from build123d import *

# Parameters (mm, degrees)
F0_R     = 2.5
F1_DEPTH = 4
F2_SIZE  = 0.5


with BuildPart() as f1:
    # F0 (on Top) → F1 (new body)
    with BuildSketch(Plane.XY):
        Polygon((4, -2.309401), (4, 2.309401), (0, 4.618802), (-4, 2.309401), (-4, -2.309401), (0, -4.618802), align=None)
        Circle(F0_R, mode=Mode.SUBTRACT)
    extrude(amount=F1_DEPTH)

    # F2
    f2_edges = [f1.edges().sort_by_distance(p)[0] for p in [
        (-2.5, 0, 4),
        (-2.5, 0, 0),
    ]]
    chamfer(f2_edges, length=F2_SIZE)


solid = f1.part
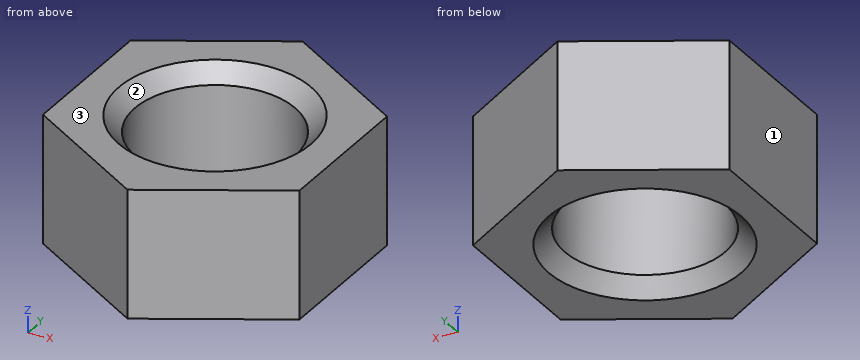
The model under review builds one solid part; all positions refer to its coordinate system, in mm. Face numbers are marked on the shaded views. Round coordinates to 2 decimals unless told otherwise and drop trailing zeros. Order: outer loops, then holes, each group sorted by start corner. A loop starts at its lowest first (then second) coordinate and runs counter-clockwise, first axis right, second up. Notation, with made-up numbers: (88, 48) -> (128, 48) arc R32 cw to (128, 80) -> close; hole circle Ø5 at (76, -19). An arc over 180 degrees is marked (long way). Use CSV: the item, a comma, the result in double quotes. Start each with the question number.
(1) Consider section B-B on z = 1.4. Write out the cut boundary in (x, y).
(2) Consider section C-C on x = 3.25. Write out the cut boundary in (y, z).
(3) Mouldability with a two-part tool opening along X and no side actions: class the marked faces 1, 2 and 3 as pulls with the +X half, pulls with the -X half, needs draft (parallel to the pull), parting line crosses it, or undercut.
(4) Consider section A-A on y = 0. Write out the cut boundary in (x, z).
(5) Wall thickness on probe 1 along X at (y, z) = (-2, 3.05); probe 2 along X at (y, z) = (-1, 3.2); probe 3 along Y at (x, z) = (-0.25, 1.2): over which ranges is each line inside the solid? List them lowest first. Write a range as from..to.
(6) Consider section D-D on y = 4. Write out the cut boundary in (x, z).
(7) Insertion check: pin 1 (1 mm diameter, centred on x = -2, z = 1, fed in from -Y); pin 2 (1 mm diameter, centred on y = 3.5, z = 0.5, fed in from +X); pin 3 (2 mm diameter, centred on x = -1, y = -1.5, fed in from +Z). Each pin has a flat end and moves straight along its axis. Give the tip position at first contact, or say it passes through.
Responses:
1,outline,"(-4, -2.31) -> (0, -4.62) -> (4, -2.31) -> (4, 2.31) -> (0, 4.62) -> (-4, 2.31) -> close; hole circle Ø5 at (0, 0)"
2,outline,"(-2.74, 0) -> (2.74, 0) -> (2.74, 4) -> (-2.74, 4) -> close"
3,face 1,"pulls with the -X half"
3,face 2,"undercut"
3,face 3,"needs draft"
4,outline,"(-4, 0) -> (-3, 0) -> (-2.5, 0.5) -> (-2.5, 3.5) -> (-3, 4) -> (-4, 4) -> close; (2.5, 0.5) -> (3, 0) -> (4, 0) -> (4, 4) -> (3, 4) -> (2.5, 3.5) -> close"
5,probe 1,"-4..-1.5, 1.5..4"
5,probe 2,"-4..-2.29, 2.29..4"
5,probe 3,"-4.47..-2.49, 2.49..4.47"
6,outline,"(-1.07, 0) -> (1.07, 0) -> (1.07, 4) -> (-1.07, 4) -> close"
7,pin 1,"y = -3.75"
7,pin 2,"x = 2.8"
7,pin 3,"z = 3.8"
